from build123d import *

# Parameters (mm, degrees)
SKETCH1_W               = 140
SKETCH1_H               = 51
BOSS_EXTRUDE1_DEPTH     = 15
CUT_EXTRUDE1_DEPTH      = 52
CUT_EXTRUDE2_DEPTH      = 1
CUT_EXTRUDE2_DEPTH_BACK = 26


with BuildPart() as part:
    # Sketch1 → Boss-Extrude1 (new body)
    with BuildSketch(Plane.XY):
        with Locations((9.063380282, 3.112676056)):
            Rectangle(SKETCH1_W, SKETCH1_H)
    extrude(amount=BOSS_EXTRUDE1_DEPTH)

    # Sketch2 → Cut-Extrude1 (cut, through all)
    with BuildSketch(Plane(origin=(0, 28.612676056, 0), x_dir=(1, 0, 0), z_dir=(0, 1, 0))):
        Polygon((74.563380282, -2.5), (74.563380282, 0), (71.563380282, 0), (71.563380282, -2.5), (71.563380282, -9.25), (76.563380282, -9.25), (76.563380282, -2.5), align=None)
    extrude(amount=-CUT_EXTRUDE1_DEPTH, mode=Mode.SUBTRACT)

    # Sketch3 → Cut-Extrude2 (cut, two sides)
    with BuildSketch(Plane(origin=(0, 28.612676056, 0), x_dir=(1, 0, 0), z_dir=(0, 1, 0))) as cut_extrude2_sk:
        Polygon((-352.539176525, 0), (-60.936619718, 0), (-53.586619718, 0), (-55.553644461, -7.34103628), (-46.319594976, -7.34103628), (-48.286619718, 0), (-123.75891502, 281.666440631), (-576.450550722, 649.359910128), (-805.230812226, 367.693469497), align=None)
    extrude(amount=CUT_EXTRUDE2_DEPTH, mode=Mode.SUBTRACT)
    extrude(cut_extrude2_sk.sketch, amount=-CUT_EXTRUDE2_DEPTH_BACK, mode=Mode.SUBTRACT)


solid = part.part
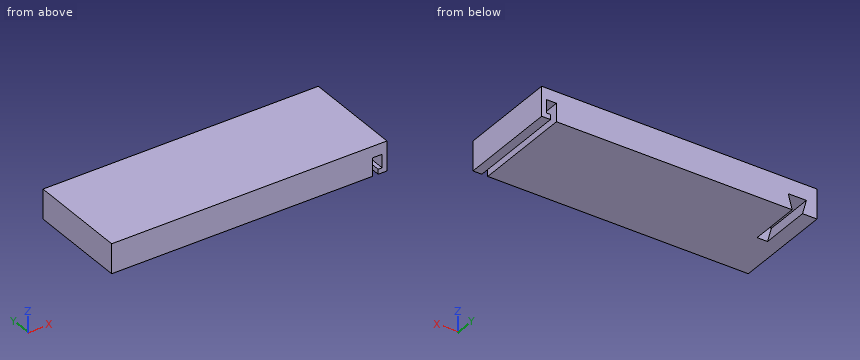
The listing builds one solid part. Answer for the finished solid, in the listing's coordinates (mm). Coordinates: 2 decimals unless noted, no trailing zeros. Write each loop counter-clockwise with the first axis right and the second up, starting at its lowest first coordinate (ties: lowest second). Pieces come first, ordered by that corner, then holes. Notation, with made-up numbers: M 64.5,69 L 96.5,69 A33 cw 96.5,107 Z; hole C -2,-7 d1. An arc over 180 degrees is marked long. Use one line per item in the form item = value.
Item 1: Find section A-A, the plane z = 6. Give the vertices of the cut face in (x, y).
Model answer:
outline = M -60.94,-22.39 L 71.56,-22.39 L 71.56,28.61 L -46.68,28.61 L -46.68,2.61 L -55.19,2.61 L -55.19,28.61 L -60.94,28.61 Z; M 76.56,-22.39 L 79.06,-22.39 L 79.06,28.61 L 76.56,28.61 Z
Item 2: Find section B-B, the plane y = 5. Give the vertices of the cut face in (x, z).
Model answer:
outline = M -60.94,0 L -53.59,0 L -55.55,7.34 L -46.32,7.34 L -48.29,0 L 71.56,0 L 71.56,9.25 L 76.56,9.25 L 76.56,2.5 L 74.56,2.5 L 74.56,0 L 79.06,0 L 79.06,15 L -60.94,15 Z
Item 3: Find section C-C, the plane y = -4.5. Give the vertices of the cut face in (x, z), plus the area to 3 significant figures.
Model answer:
outline = M -60.94,0 L 71.56,0 L 71.56,9.25 L 76.56,9.25 L 76.56,2.5 L 74.56,2.5 L 74.56,0 L 79.06,0 L 79.06,15 L -60.94,15 Z
area = 2,060 mm2
Item 4: Find the intervals of material crossed by probe 1 along X at (y, z) = (-3, 6.25); probe 2 along X at (y, z) = (25, 1); probe 3 along X at (y, z) = (21.5, 6.25), in increasing order.
Model answer:
probe_1 = -60.94 to 71.56, 76.56 to 79.06
probe_2 = -60.94 to -53.85, -48.02 to 71.56, 74.56 to 79.06
probe_3 = -60.94 to -55.26, -46.61 to 71.56, 76.56 to 79.06
